```python
from build123d import *

# Parameters (mm, degrees)
F1_DEPTH    = 74.9545320868
F2_R        = 8.1435947288
F3_DEPTH    = 124.2861971259
F5_R        = 11.2476479719
F6_DEPTH    = 38.057185469
F7_T1_DEPTH = 183.0316575771


# Not quite as in the source:
# - a fillet or chamfer that OpenCascade refuses, or shapes differently, is made with other operations: its cross-section is extruded or revolved along the edge and cut away or added


with BuildPart() as f1:
    # F0 (on Top) → F1 (new body)
    with BuildSketch(Plane.XY):
        Polygon((26.3189487159, 57.2941713035), (-16.4525061846, 57.2941713035), (-17.4609050155, 56.2243200839), (-4.0535703301, 19.2379858345), (28.3696912229, 25.376688689), align=None)
    extrude(amount=F1_DEPTH)

    # F2 (on face) → F3 (cut)
    with BuildSketch(Plane.XY.offset(74.9545320868)):
        with Locations((12.1580604464, 43.6755083501)):
            Circle(F2_R)
    extrude(amount=-F3_DEPTH, mode=Mode.SUBTRACT)

    # F5 (on face) → F6 (cut, through all)
    with BuildSketch(Plane(origin=(0, 57.2941713035, 0), x_dir=(-1, 0, 0), z_dir=(0, 1, 0))):
        with Locations((-9.5685087144, 45.682426542)):
            Circle(F5_R)
    extrude(amount=-F6_DEPTH, mode=Mode.SUBTRACT)

    # F7: fillet of radius 25.4 on 1 edges, made by hand

    # F7_s2 → F7_t1 (cut)
    with BuildSketch(Plane.XY.offset(-54.0385627451)):
        with BuildLine():
            ThreePointArc((17.1845559853, 23.2590047077), (-0.1162411856, 26.147331869), (-11.4199898846, 39.559463761))
            Line((-11.4199898846, 39.559463761), (-4.0535703301, 19.2379858345))
            Line((-4.0535703301, 19.2379858345), (17.1845559853, 23.2590047077))
        make_face()
    extrude(amount=F7_T1_DEPTH, mode=Mode.SUBTRACT)


solid = f1.part
```
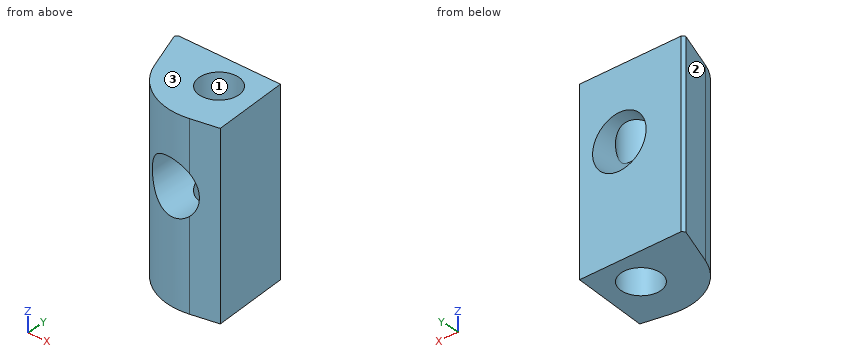
The listing builds one solid part. Answer for the finished solid, in the listing's coordinates (mm). Face numbers are marked on the shaded views. Give positions to 0.01 mm unless a question says otherwise; leave off trailing zeros. Order: outer loops, then holes, each group sorted by start corner. A loop starts at its lowest first (then second) coordinate and runs counter-clockwise, first axis right, second up. Notation, with made-up numbers: (87.5, 29) -> (139.5, 29) arc R8 cw to (139.5, 39) -> close; hole circle Ø4 at (3, 31.25). An arc over 180 degrees is marked (long way). Answer as a JSON object with one key per item and string values. Group by question number.
Item 1: The part is cut by section D-D on y = 28.5. Write down the section's boundary in (x, z).
Item 2: Flat-ended cylindrical pins translate along their axes: pin 1 (2 mm diameter, centred on y = 31.5, z = 60.5, fed in from -X); pin 2 (1 mm diameter, centred on y = 49.5, z = 30, fed in from +X); pin 3 (13 mm diameter, centred on x = 12.16, y = 43.68, fed in from +Z); pin 4 (3 mm diameter, centred on y = 48, z = 52.5, fed in from -X). Find the tip coordinate at first contact, or state that the pin passes through.
Item 3: The part is cut by section A-A on y = 44.5. Write down the section's boundary in (x, z), and give its area (3 significant figures).
Item 4: Determine the mould class of the marked faces 1, 2 and 3 for opening direction Y: pulls with the +Y half, pulls with the -Y half, needs draft (parallel to the pull), parting line crosses it, or undercut.
Item 5: The part is cut by section C-C on x = 13.5. Write down the section's boundary in (y, z).
Item 6: The part is cut by section B-B on z = 64. Write down the section's boundary in (x, y), and give its area (3 significant figures).
Item 7: Consider L1, parallel to Z at x = 3, y = 36; L2, parallel to X at y = 49, z = 17; L3, parallel to X at y = 45, z = 43.5. Determine where each line is inside the solid, lowest interval first. Write a range as from..to.
Result set:
{
 "1": {"outline": "(-3.55, 0) -> (28.17, 0) -> (28.17, 74.95) -> (-3.55, 74.95) -> close; hole circle Ø22.5 at (9.57, 45.68)"},
 "2": {"pin 1": "x = -7.49", "pin 2": "x = 26.85", "pin 3": "through", "pin 4": "x = -15.02"},
 "3": {"outline": "(-13.21, 0) -> (4.06, 0) -> (4.06, 35.88) arc R11.25 cw to (4.06, 55.49) -> (4.06, 74.95) -> (-13.21, 74.95) -> close; (20.26, 0) -> (27.14, 0) -> (27.14, 74.95) -> (20.26, 74.95) -> (20.26, 49.18) arc R11.25 cw to (20.26, 42.19) -> close", "area": "1,730 mm²"},
 "4": {"face 1": "undercut", "face 2": "pulls with the -Y half", "face 3": "needs draft"},
 "5": {"outline": "(22.84, 0) -> (35.64, 0) -> (35.64, 35.14) -> (22.84, 35.14) -> close; (22.84, 56.22) -> (35.64, 56.22) -> (35.64, 74.95) -> (22.84, 74.95) -> close; (51.71, 0) -> (57.29, 0) -> (57.29, 35.14) -> (51.71, 35.14) -> close; (51.71, 56.22) -> (57.29, 56.22) -> (57.29, 74.95) -> (51.71, 74.95) -> close"},
 "6": {"outline": "(-17.46, 56.22) -> (-11.42, 39.56) arc R25.4 ccw to (17.18, 23.26) -> (28.37, 25.38) -> (26.32, 57.29) -> (-16.45, 57.29) -> close; hole circle Ø16.29 at (12.16, 43.68)", "area": "1,060 mm²"},
 "7": {"L1": "0..36.55, 54.81..74.95", "L2": "-14.84..6, 18.32..26.85", "L3": "-13.39..-1.47, 20.6..27.11"}
}
